Build history of the part. All positions in model axes, mm. A direction names the side the tool comes from. Round coordinates to 2 decimals unless told otherwise and drop trailing zeros. Order: outer loops, then holes, each group sorted by start corner. A loop starts at its lowest first (then second) coordinate and runs counter-clockwise, first axis right, second up. Notation, with made-up numbers: M -5.75,-15 L 51.25,-15 A25 ccw 51.25,23 Z; hole C 24.25,85.5 d10. An arc over 180 degrees is marked long. One line per item, written item: value. Start each with the question number.
Item 1: Two-plate mould, pull along Y, no slides. Class faces 1 (the flat face through (-5.2, -26.812, 5.2)), 2 (the conical face through (-5.18, 18.51, -1.15)), 3 (the flat face through (-8, -4.933, 0)): +Y half, -Y half, draft (parallel to the pull), parting line (faces both ways), or undercut.
Item 2: Pin check, flat tips, straight feed: pin 1 (8 mm diameter, centred on y = -8, z = -22.5, fed in from +X); pin 2 (2 mm diameter, centred on x = 11.5, z = 12, fed in from -Y); pin 3 (12 mm diameter, centred on x = -4.5, z = 4, fed in from +Y). Stop position of each tip, or through.
Item 3: Tool access for faces 4 (the flat face through (-6, 5.496, 6)), 5 (the cylindrical face through (2.13, -40.68, 6.76)): list every direction of +Z, -Z, +X, -X, +Y, -Y with a clear straight run to the whole face (end or side of a thin tool).
Item 4: Band-saw the part on A-A, the plane y = -40.5. Write the cut outline in (x, z), then the cut area to 3 significant figures.
Item 5: Band-saw the part on B-B, the plane y = 1. Write the cut outline in (x, z), then the cut area to 3 significant figures.
Item 6: Probe L1, parallel to Y at x = -17, z = 8.5; L2, parallel to Y at x = 6.5, z = 9.5; L3, parallel to Y at x = 10, z = -1. List the from-to ranges inside material, lowest first.
```python
from build123d import *

# Parameters (mm, degrees)
F2_W = 54.9414514213
F2_H = 7.087636739


with BuildPart() as f1:
    # F0 (on Right) → F1 (revolve)
    with BuildSketch(Plane.YZ):
        with BuildLine():
            Line((-26.8122032285, 25.1458510756), (-26.8122032285, 0))
            Line((-26.8122032285, 0), (0, 0))
            Line((0, 0), (27.0384699106, 0))
            Line((27.0384699106, 0), (5.4959878325, 13.4000256658))
            Line((5.4959878325, 13.4000256658), (5.4959878325, 7.5829699636))
            Line((5.4959878325, 7.5829699636), (-4.9333125353, 7.7540650964))
            Line((-4.9333125353, 7.7540650964), (-4.9333125353, 18.4741187841))
            ThreePointArc((-4.9333125353, 18.4741187841), (-13.4024776279, 29.9108782654), (-26.8122032285, 25.1458510756))
        make_face()
    revolve(axis=Axis((0, -13.4061016142, 0), (0, 1, 0)))

    # F2 (on Right) → F3 (revolve)
    with BuildSketch(Plane.YZ):
        with Locations((-27.4707257106, 3.5438183695)):
            Rectangle(F2_W, F2_H)
        Polygon((-54.9414514213, 0), (-54.9414514213, 7.087636739), (-76.563516876, 0), align=None)
    revolve(axis=Axis((0, -27.4707257106, 0), (0, 1, 0)))


solid = f1.part
```
Output:
1. face 1: -Y half
1. face 2: +Y half
1. face 3: undercut
2. pin 1: stops at x = 21.02
2. pin 2: stops at y = -26.81
2. pin 3: stops at y = 27
3. face 4: none
3. face 5: -Y
4. outline: C 0,0 d14.18
4. area: 158 mm²
5. outline: C 0,0 d15.31
5. area: 184 mm²
6. L1: y = -26.81 to -4.95
6. L2: y = -26.81 to -4.93, 5.5 to 8.53
6. L3: y = -26.81 to -4.93, 5.5 to 10.88
